Source: CAD feature listing. Evaluate the final solid. Frame: model axes, mm. Face numbers are marked on the shaded views. A direction names the side the tool comes from. Give positions to 0.01 mm unless a question says otherwise; leave off trailing zeros. Order: outer loops, then holes, each group sorted by start corner. A loop starts at its lowest first (then second) coordinate and runs counter-clockwise, first axis right, second up. Notation, with made-up numbers: M -18,30.5 L -12,30.5 A18 ccw -12,56.5 Z; hole C 76.25,7.25 d7. An arc over 180 degrees is marked long. Answer as a JSON object with one key per item and string values. Group by question number.
1. Section query B-B (x = -35). Output: boundary loops of the cut face in (y, z), plus the area to 3 significant figures.
2. Pin query (flat end, axial travel): P1, Ø1.5, axis at x = -43.5, y = -124, coming from the -Z side; P2, Ø5, axis at y = -129.5, z = -272, coming from the +X side; P3, Ø12.5, axis at x = 0, y = -100, coming from the +Z side; P4, Ø18, axis at x = 0, y = -150, coming from the -Z side. Return the tip coordinate at first contact, or that it passes through.
3. Section query A-A (z = -271.5). Output: boundary loops of the cut face in (x, y), plus the area to 3 significant figures.
4. Set-up query: the marked faces 4, 5 and 6. Return all of +Z, -Z, +X, -X, +Y, -Y with unobstructed straight access to the full face (end or side cutting, diameter ignored); none if empty.
5. Pull-direction query (X, two-part tool) for the marked faces 1, 2 and 3; classes: +X half, -X half, draft (parallel to the pull), parting line (faces both ways), or undercut.
6. Section query D-D (y = -82.5). Output: boundary loops of the cut face in (x, z).
7. Material intervals for L1, parallel to Z at x = -89.5, y = -150; L2, parallel to Z at x = -5.5, y = -117; L3, parallel to X at y = -73, z = -259.5, sorted ascending. Write a range as [from, to].
8. Section query C-C (z = -224). Output: boundary loops of the cut face in (x, y).
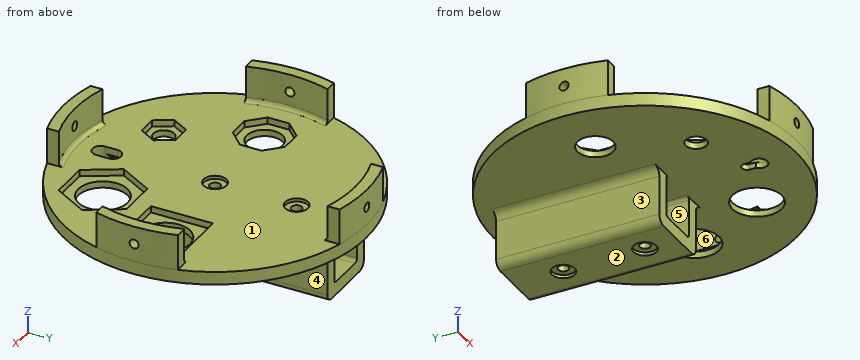
from build123d import *

# Parameters (mm, degrees)
SKETCH159_R       = 7
EXTRUDE060_DEPTH  = 2
SKETCH158_R       = 7
EXTRUDE059_DEPTH  = 2
SKETCH143_R       = 3.2
EXTRUDE044_DEPTH  = 50
SKETCH157_W       = 38
SKETCH157_H       = 38
EXTRUDE058_DEPTH  = 10
EXTRUDE036_DEPTH  = 100
EXTRUDE020_DEPTH  = 10
CYLINDER133_R     = 2.8
CYLINDER133_DEPTH = 300
CYLINDER134_R     = 2.8
CYLINDER134_DEPTH = 300
EXTRUDE023_DEPTH  = 30
SKETCH037_R       = 93
SKETCH037_R_2     = 11
SKETCH037_R_3     = 15.1
SKETCH037_R_4     = 6.4
EXTRUDE019_DEPTH  = 8
FILLET028_R       = 2
FILLET029_R       = 5
FILLET030_R       = 2.5


with BuildPart() as extrude060:
    # Sketch159 → Extrude060 (new body)
    with BuildSketch(Plane.XY.offset(-244)):
        with Locations((0, -100)):
            Circle(SKETCH159_R)
        with Locations((0, -150)):
            Circle(SKETCH159_R)
    extrude(amount=EXTRUDE060_DEPTH)


with BuildPart() as extrude060_1:
    # Extrude060 placement: moved
    add(extrude060.part.moved(Location((0, 0, -40))))


with BuildPart() as tslotcuts:
    # Sketch158 → Extrude059 (new body)
    with BuildSketch(Plane.XY.offset(-244)):
        with Locations((0, -100)):
            Circle(SKETCH158_R)
        with Locations((0, -150)):
            Circle(SKETCH158_R)
    extrude(amount=EXTRUDE059_DEPTH)

    # Fusion135: union Extrude060
    add(extrude060_1.part)


with BuildPart() as extrude044:
    # Sketch143 → Extrude044 (new body)
    with BuildSketch(Plane.XY):
        with Locations((0, -150)):
            Circle(SKETCH143_R)
        with Locations((0, -100)):
            Circle(SKETCH143_R)
    extrude(amount=EXTRUDE044_DEPTH)


with BuildPart() as extrude044_1:
    # Extrude044 placement: moved
    add(extrude044.part.moved(Location((0, 0, -290))))


with BuildPart() as level5cuts002:
    # Sketch157 → Extrude058 (new body)
    with BuildSketch(Plane.XY):
        with Locations((57, -150)):
            Rectangle(SKETCH157_W, SKETCH157_H)
        Polygon((-29, -210.392305), (-23, -200), (-29, -189.607695), (-41, -189.607695), (-47, -200), (-41, -210.392305), align=None)
        Polygon((47, -220.78461), (59, -200), (47, -179.21539), (23, -179.21539), (11, -200), (23, -220.78461), align=None)
        Polygon((-50.372583, -166), (-41, -156.627417), (-41, -143.372583), (-50.372583, -134), (-63.627417, -134), (-73, -143.372583), (-73, -156.627417), (-63.627417, -166), align=None)
    extrude(amount=EXTRUDE058_DEPTH)


with BuildPart() as level5cuts002_1:
    # Extrude058 placement: moved
    add(level5cuts002.part.moved(Location((0, 0, -246))))

    # Fusion133: union Extrude044
    add(extrude044_1.part)

    # Fusion136: union tSlotCuts
    add(tslotcuts.part)


with BuildPart() as level5s012:
    # Sketch054 → Extrude036 (new body)
    with BuildSketch(Plane.XZ):
        Polygon((-21, -250), (-13, -250), (-13, -276), (13, -276), (13, -250), (21, -250), (21, -284), (-21, -284), align=None)
    extrude(amount=EXTRUDE036_DEPTH)


with BuildPart() as level5s012_1:
    # Extrude036 placement: moved
    add(level5s012.part.moved(Location((0, -70, 0))))


with BuildPart() as obj1:
    # Sketch038 → Extrude020 (new body)
    with BuildSketch(Plane.XY):
        with BuildLine():
            ThreePointArc((-5, -220), (0, -225), (5, -220))
            Line((5, -220), (5, -212.5))
            ThreePointArc((5, -212.5), (0, -207.5), (-5, -212.5))
            Line((-5, -212.5), (-5, -220))
        make_face()
    extrude(amount=EXTRUDE020_DEPTH)


with BuildPart() as obj1_1:
    # Extrude020 placement: moved
    add(obj1.part.moved(Location((0, 0, -246.5))))


with BuildPart() as cylinder133:
    # Cylinder133 → Cylinder133 (new body)
    with BuildSketch(Plane(origin=(0, 0, 90), x_dir=(1, 0, 0), z_dir=(0, -1, 0))):
        Circle(CYLINDER133_R)
    extrude(amount=CYLINDER133_DEPTH)


with BuildPart() as m4heatsetcuts001:
    # Cylinder134 → Cylinder134 (new body)
    with BuildSketch(Plane(origin=(-150, -150, 90), x_dir=(0, 1, 0), z_dir=(1, 0, 0))):
        Circle(CYLINDER134_R)
    extrude(amount=CYLINDER134_DEPTH)

    # Fusion085: union Cylinder133
    add(cylinder133.part)


with BuildPart() as m4heatsetcuts001_1:
    # Fusion085 placement: moved
    add(m4heatsetcuts001.part.moved(Location((0, 0, -321))))


with BuildPart() as obj2:
    # Sketch041 → Extrude023 (new body)
    with BuildSketch(Plane.XY):
        with BuildLine():
            ThreePointArc((-89.576783, -125), (-93, -150), (-89.576783, -175))
            Line((-89.576783, -175), (-82.286086, -175))
            ThreePointArc((-82.286086, -125), (-86, -150), (-82.286086, -175))
            Line((-89.576783, -125), (-82.286086, -125))
        make_face()
        with BuildLine():
            ThreePointArc((25, -60.423217), (0, -57), (-25, -60.423217))
            Line((-25, -60.423217), (-25, -67.713914))
            ThreePointArc((25, -67.713914), (0, -64), (-25, -67.713914))
            Line((25, -60.423217), (25, -67.713914))
        make_face()
        with BuildLine():
            ThreePointArc((89.576783, -175), (93, -150), (89.576783, -125))
            Line((89.576783, -125), (82.286086, -125))
            ThreePointArc((82.286086, -175), (86, -150), (82.286086, -125))
            Line((89.576783, -175), (82.286086, -175))
        make_face()
        with BuildLine():
            ThreePointArc((-25, -239.576783), (0, -243), (25, -239.576783))
            Line((25, -239.576783), (25, -232.286086))
            ThreePointArc((-25, -232.286086), (0, -236), (25, -232.286086))
            Line((-25, -239.576783), (-25, -232.286086))
        make_face()
    extrude(amount=EXTRUDE023_DEPTH)


with BuildPart() as obj2_1:
    # Extrude023 placement: moved
    add(obj2.part.moved(Location((0, 0, -250))))


with BuildPart() as level5s015:
    # Sketch037 → Extrude019 (new body)
    with BuildSketch(Plane.XY):
        with Locations((0, -150)):
            Circle(SKETCH037_R)
        with Locations((-57, -150)):
            Circle(SKETCH037_R_2, mode=Mode.SUBTRACT)
        with Locations((57, -150)):
            Circle(SKETCH037_R_3, mode=Mode.SUBTRACT)
        with Locations((35, -200)):
            Circle(SKETCH037_R_3, mode=Mode.SUBTRACT)
        with Locations((-35, -200)):
            Circle(SKETCH037_R_4, mode=Mode.SUBTRACT)
        with BuildLine():
            ThreePointArc((-3.2, -216.158125), (0, -225), (3.2, -216.158125))
            Line((3.2, -216.158125), (3.2, -212.5))
            ThreePointArc((3.2, -212.5), (0, -209.3), (-3.2, -212.5))
            Line((-3.2, -212.5), (-3.2, -216.158125))
        make_face(mode=Mode.SUBTRACT)
    extrude(amount=EXTRUDE019_DEPTH)


with BuildPart() as level5s015_1:
    # Extrude019 placement: moved
    add(level5s015.part.moved(Location((0, 0, -250))))

    # Fusion083: union obj2
    add(obj2_1.part)

    # Cut035: cut m4HeatSetCuts001
    add(m4heatsetcuts001_1.part, mode=Mode.SUBTRACT)

    # Cut041: cut obj1
    add(obj1_1.part, mode=Mode.SUBTRACT)

    # Fusion134: union level5s012
    add(level5s012_1.part)

    # Cut098: cut level5Cuts002
    add(level5cuts002_1.part, mode=Mode.SUBTRACT)

    # Fillet028
    fillet028_edges = [level5s015_1.edges().sort_by_distance(p)[0] for p in [
        (-13, -120, -250),
        (13, -120, -250),
        (-13, -120, -276),
        (13, -120, -276),
    ]]
    fillet(fillet028_edges, radius=FILLET028_R)

    # Fillet029
    fillet029_edges = [level5s015_1.edges().sort_by_distance(p)[0] for p in [
        (-21, -120, -250),
        (21, -120, -250),
        (-21, -120, -284),
        (21, -120, -284),
    ]]
    fillet(fillet029_edges, radius=FILLET029_R)

    # Fillet030
    fillet030_edges = [level5s015_1.edges().sort_by_distance(p)[0] for p in [
        (86, -150, -242),
        (0, -64, -242),
        (0, -236, -242),
        (-86, -150, -242),
    ]]
    fillet(fillet030_edges, radius=FILLET030_R)


solid = level5s015_1.part
Answer sheet:
{
 "1": {"outline": "M -236.16,-250 L -206.4,-250 L -206.4,-246 L -210.39,-246 L -210.39,-242 L -236.16,-242 Z; M -193.6,-250 L -63.84,-250 L -63.84,-242 L -189.61,-242 L -189.61,-246 L -193.6,-246 Z", "area": "1,240 mm^2"},
 "2": {"P1": "z = -250", "P2": "x = 21", "P3": "z = -244", "P4": "z = -284"},
 "3": {"outline": "M -21,-170 L -13,-170 L -13,-70 L -21,-70 Z; M 13,-170 L 21,-170 L 21,-70 L 13,-70 Z", "area": "1,600 mm^2"},
 "4": {"face 4": "-Z, +X, +Y, -Y", "face 5": "+Y, -Y", "face 6": "+Z"},
 "5": {"face 1": "undercut", "face 2": "draft", "face 3": "-X half"},
 "6": {"outline": "M -63.97,-250 L -26,-250 A5 cw -21,-255 L -21,-279 A5 ccw -16,-284 L 16,-284 A5 ccw 21,-279 L 21,-255 A5 cw 26,-250 L 63.97,-250 L 63.97,-242 L -63.97,-242 Z; hole M -13,-274 A2 ccw -11,-276 L 11,-276 A2 ccw 13,-274 L 13,-252 A2 ccw 11,-250 L -11,-250 A2 ccw -13,-252 Z"},
 "7": {"L1": "[-250, -233.8], [-228.2, -220]", "L2": "[-284, -276], [-250, -242]", "L3": "[-21, -13], [13, 21]"},
 "8": {"outline": "M -89.58,-175 L -82.29,-175 A86 cw -82.29,-125 L -89.58,-125 A93 ccw Z; M -25,-239.58 A93 ccw 25,-239.58 L 25,-232.29 A86 cw -25,-232.29 Z; M -25,-67.71 A86 cw 25,-67.71 L 25,-60.42 A93 ccw -25,-60.42 Z; M 82.29,-175 L 89.58,-175 A93 ccw 89.58,-125 L 82.29,-125 A86 cw Z"}
}
